Source: CAD feature listing. Evaluate the final solid. Frame: model axes, mm. Give positions to 0.01 mm unless a question says otherwise; leave off trailing zeros. Write each loop counter-clockwise with the first axis right and the second up, starting at its lowest first coordinate (ties: lowest second). Pieces come first, ordered by that corner, then holes. Notation, with made-up numbers: (75, 86) -> (123, 86) arc R17 cw to (123, 101) -> close; hole circle Ø1 at (75, -2). An arc over 180 degrees is marked (long way). Write item = value, one per line.
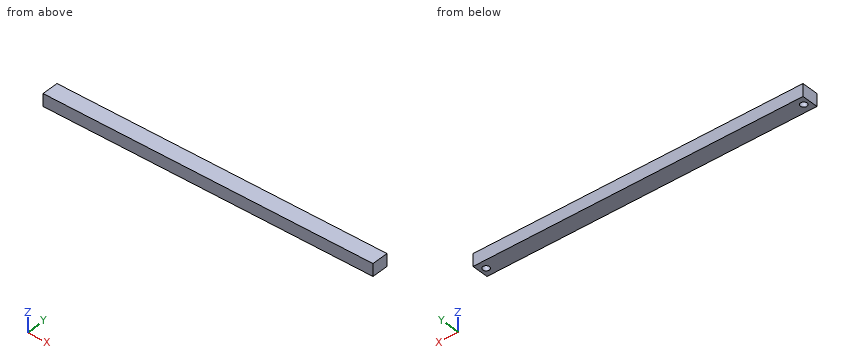
from build123d import *

# Parameters (mm, degrees)
SKETCH1_W           = 400
SKETCH1_H           = 20
BOSS_EXTRUDE1_DEPTH = 7.5
SKETCH2_R           = 4
CUT_EXTRUDE1_DEPTH  = 10


with BuildPart() as part:
    # Sketch1 → Boss-Extrude1 (new body, symmetric)
    with BuildSketch(Plane.XY):
        Rectangle(SKETCH1_W, SKETCH1_H)
    extrude(amount=BOSS_EXTRUDE1_DEPTH, both=True)

    # Sketch2 → Cut-Extrude1 (cut)
    with BuildSketch(Plane(origin=(0, 0, -7.5), x_dir=(-1, 0, 0), z_dir=(0, 0, -1))):
        with Locations((-192.5, 0)):
            Circle(SKETCH2_R)
    cut_extrude1 = extrude(amount=-CUT_EXTRUDE1_DEPTH, mode=Mode.SUBTRACT)

    # Mirror1: Cut-Extrude1 across plane
    add(cut_extrude1.mirror(Plane(origin=(0, 0, 0), x_dir=(0, 0, 1), z_dir=(1, 0, 0))), mode=Mode.SUBTRACT)


solid = part.part
1) Cut plane B-B (y = 0). Return the cut outline in (x, z), then the cut area to 3 significant figures.
Computed:
outline = (-200, -7.5) -> (-196.5, -7.5) -> (-196.5, 2.5) -> (-188.5, 2.5) -> (-188.5, -7.5) -> (188.5, -7.5) -> (188.5, 2.5) -> (196.5, 2.5) -> (196.5, -7.5) -> (200, -7.5) -> (200, 7.5) -> (-200, 7.5) -> close
area = 5,840 mm²
2) Cut plane A-A (x = 192.5). Return the cut outline in (y, z), then the cut area to 3 significant figures.
Computed:
outline = (-10, -7.5) -> (-4, -7.5) -> (-4, 2.5) -> (4, 2.5) -> (4, -7.5) -> (10, -7.5) -> (10, 7.5) -> (-10, 7.5) -> close
area = 220 mm²
3) Material intervals for L1, parallel to Y at x = 192.5, z = -1, sorted ascending.
Computed:
L1 = -10 to -4, 4 to 10
4) Contact query for flat-ended pins moving along their axis: pin 1 (4 mm diameter, centred on x = 191, y = -1.5, fed in from -Z); pin 2 (4 mm diameter, centred on x = -191.5, y = -0.5, fed in from -Z). Output: stop coordinate, or through.
Computed:
pin_1 = -7.5
pin_2 = 2.5
